Part model, mm, in its own coordinate system. Give positions to 0.01 mm unless a question says otherwise; leave off trailing zeros. Write each loop counter-clockwise with the first axis right and the second up, starting at its lowest first coordinate (ties: lowest second). Pieces come first, ordered by that corner, then holes.
```python
from build123d import *

# Parameters (mm, degrees)
F0_R     = 21.3676548909
F1_DEPTH = 0.635


with BuildPart() as f1:
    # F0 (on Front) → F1 (new body)
    with BuildSketch(Plane.XZ):
        with BuildLine():
            Line((68.9142415212, 26.0405766578), (0, 26.0405766578))
            Line((0, 26.0405766578), (-68.9142415212, 26.0405766578))
            Line((-68.9142415212, 26.0405766578), (-68.9142415212, 11.925470218))
            add(Edge.make_bspline(
                [(-68.9142415212, 11.925470218), (-58.5539967516, 7.5661347342), (-38.6011677749, -0.8164003994), (-24.1054599416, -13.5221086271), (-17.1279080613, -19.6149534313)],
                knots=[0, 0, 0, 0, 0.5194376377, 1, 1, 1, 1], degree=3))
            ThreePointArc((-17.1279080613, -19.6149534313), (0, -26.0405766578), (17.1279080613, -19.6149534313))
            add(Edge.make_bspline(
                [(68.9142415212, 11.925470218), (58.5539967516, 7.5661347342), (38.6011677749, -0.8164003994), (24.1054599416, -13.5221086271), (17.1279080613, -19.6149534313)],
                knots=[0, 0, 0, 0, 0.5194376377, 1, 1, 1, 1], degree=3))
            Line((68.9142415212, 11.925470218), (68.9142415212, 26.0405766578))
        make_face()
        Circle(F0_R, mode=Mode.SUBTRACT)
    extrude(amount=F1_DEPTH)


solid = f1.part
```
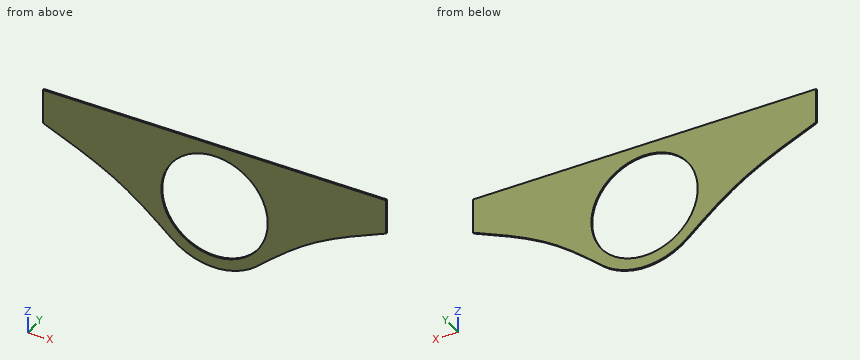
1) Saw through at C-C, the plane z = -23. Write the cut outline in (x, y) (3 decimals), then the cut area to 3 significant figures.
Answers follow:
outline: (-12.211, -0.635) - (12.211, -0.635) - (12.211, 0) - (-12.211, 0) - close
area: 15.5 mm2
2) Saw through at B-B, the plane z = 16. Write the cut outline in (x, y) (1 decimal).
Answers follow:
outline: (-68.9, -0.6) - (-14.2, -0.6) - (-14.2, 0) - (-68.9, 0) - close; (14.2, -0.6) - (68.9, -0.6) - (68.9, 0) - (14.2, 0) - close
3) Saw through at A-A, the plane x = 0. Write the cut outline in (y, z) (3 decimals), then the cut area to 3 significant figures.
Answers follow:
outline: (-0.635, -26.041) - (0, -26.041) - (0, -21.368) - (-0.635, -21.368) - close; (-0.635, 21.368) - (0, 21.368) - (0, 26.041) - (-0.635, 26.041) - close
area: 5.93 mm2
4) Wall check: L1, parallel to X at y = -0.45, z = 15; L2, parallel to X at y = -0.3, z = -13; L3, parallel to Z at x = 6, y = -0.1. Give the ranges that are in metal, low to high.
Answers follow:
L1: x = -68.91 to -15.22, 15.22 to 68.91
L2: x = -24.81 to -16.96, 16.96 to 24.81
L3: z = -25.34 to -20.51, 20.51 to 26.04
